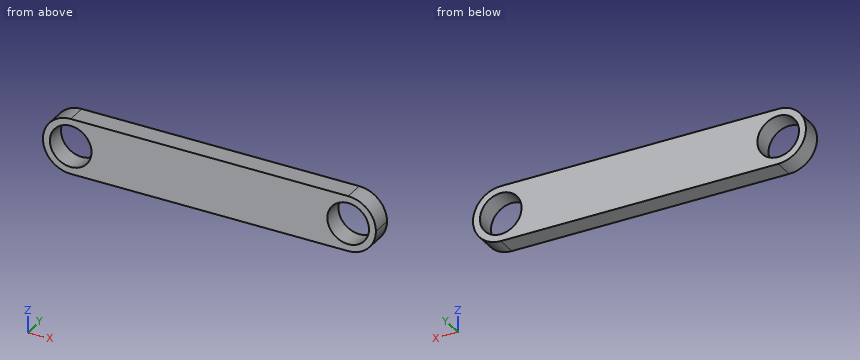
```python
from build123d import *

# Parameters (mm, degrees)
F0_R     = 4.7625
F1_DEPTH = 4.572


with BuildPart() as f1:
    # F0 (on Front) → F1 (new body)
    with BuildSketch(Plane.XZ):
        with BuildLine():
            ThreePointArc((-31.75, -6.35), (-27.259872, -4.490128), (-25.4, 0))
            ThreePointArc((-25.4, 0), (-27.259872, 4.490128), (-31.75, 6.35))
            ThreePointArc((-31.75, 6.35), (-38.1, 0), (-31.75, -6.35))
        make_face()
        with Locations((-31.75, 0)):
            Circle(F0_R, mode=Mode.SUBTRACT)
        with BuildLine():
            ThreePointArc((-31.75, 6.35), (-27.259872, 4.490128), (-25.4, 0))
            ThreePointArc((-25.4, 0), (-27.259872, -4.490128), (-31.75, -6.35))
            Line((-31.75, -6.35), (31.75, -6.35))
            ThreePointArc((31.75, -6.35), (25.4, 0), (31.75, 6.35))
            Line((31.75, 6.35), (-31.75, 6.35))
        make_face()
        with BuildLine():
            ThreePointArc((38.1, 0), (36.240128, 4.490128), (31.75, 6.35))
            ThreePointArc((31.75, 6.35), (25.4, 0), (31.75, -6.35))
            ThreePointArc((31.75, -6.35), (36.240128, -4.490128), (38.1, 0))
        make_face()
        with Locations((31.75, 0)):
            Circle(F0_R, mode=Mode.SUBTRACT)
    extrude(amount=F1_DEPTH)


solid = f1.part
```
Input: part model. Units: mm. Frame: model coordinates. Round coordinates to 2 decimals unless told otherwise and drop trailing zeros. Write each loop counter-clockwise with the first axis right and the second up, starting at its lowest first coordinate (ties: lowest second). Pieces come first, ordered by that corner, then holes. Notation, with made-up numbers: M -17,75.25 L -13,75.25 A29 cw -13,108.25 Z; hole C 44,53.5 d10. An arc over 180 degrees is marked long. Write each question's results on one line, items separated by ' | '.
Q1. Section query A-A (y = -1.65). State how many separate pieces and enclosed holes the cut face has, and give its area (3 significant figures).
Results:
separate pieces: 1 | enclosed holes: 2 | area: 791 mm^2
Q2. Pin query (flat end, axial travel): P1, Ø1.5, axis at y = -1, z = 5, coming from the +X side; P2, Ø1.5, axis at y = -4, z = -4.5, coming from the -X side. Return the tip coordinate at first contact, or that it passes through.
Results:
P1: stops at x = 36.47 | P2: stops at x = -36.87
Q3. Line query: line 1 along X through (y, z) = (-0.3, 4.25); line 2 along X through (y, z) = (-0.65, 3.25); line 3 along Z through (x, y) = (31.75, -2.75). Output: solid intervals per line, ascending.
Results:
line 1: x = -36.47 to -33.9, -29.6 to 29.6, 33.9 to 36.47 | line 2: x = -37.21 to -35.23, -28.27 to 28.27, 35.23 to 37.21 | line 3: z = -6.35 to -4.76, 4.76 to 6.35
Q4. Section query B-B (z = -3). Return loops of the section in (x, y), and give its area (3 significant figures).
Results:
outline: M -37.35,-4.57 L -35.45,-4.57 L -35.45,0 L -37.35,0 Z; M -28.05,-4.57 L 28.05,-4.57 L 28.05,0 L -28.05,0 Z; M 35.45,-4.57 L 37.35,-4.57 L 37.35,0 L 35.45,0 Z | area: 274 mm^2
Q5. Section query C-C (z = 2.5). Return loops of the section in (x, y), and give its area (3 significant figures).
Results:
outline: M -37.59,-4.57 L -35.8,-4.57 L -35.8,0 L -37.59,0 Z; M -27.7,-4.57 L 27.7,-4.57 L 27.7,0 L -27.7,0 Z; M 35.8,-4.57 L 37.59,-4.57 L 37.59,0 L 35.8,0 Z | area: 270 mm^2
